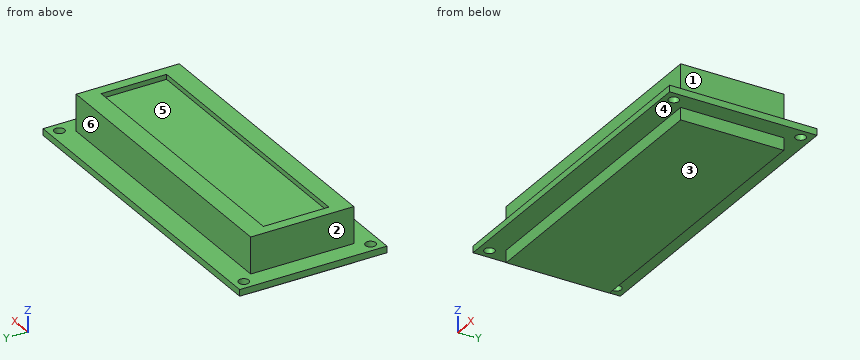
```python
from build123d import *

# Parameters (mm, degrees)
SKETCH2_W           = 80
SKETCH2_H           = 36
SKETCH2_W_2         = 71
SKETCH2_H_2         = 25.2
SKETCH2_W_3         = 66
SKETCH2_H_3         = 16
BOSS_EXTRUDE1_DEPTH = 1.6
BOSS_EXTRUDE2_START = 8.9
SKETCH2_3_W         = 71
SKETCH2_3_H         = 25.2
SKETCH2_3_W_2       = 66
SKETCH2_3_H_2       = 16
BOSS_EXTRUDE2_DEPTH = 13.5
CUT_EXTRUDE1_START  = 8.9
SKETCH2_4_W         = 66
SKETCH2_4_H         = 16
CUT_EXTRUDE1_DEPTH  = 1.2
SKETCH3_R           = 1.25
CUT_EXTRUDE2_DEPTH  = 45.757234052


with BuildPart() as part:
    # Sketch2 → Boss-Extrude1 (new body)
    # profile 1 of 3: a face of its own
    with BuildSketch(Plane.XY):
        Rectangle(SKETCH2_W, SKETCH2_H)
        Rectangle(SKETCH2_W_2, SKETCH2_H_2, mode=Mode.SUBTRACT)
    # profile 2 of 3: a face of its own
    with BuildSketch(Plane.XY):
        Rectangle(SKETCH2_W_2, SKETCH2_H_2)
        Rectangle(SKETCH2_W_3, SKETCH2_H_3, mode=Mode.SUBTRACT)
    # profile 3 of 3: a face of its own
    with BuildSketch(Plane.XY):
        Rectangle(SKETCH2_W_3, SKETCH2_H_3)
    extrude(amount=-BOSS_EXTRUDE1_DEPTH)

    # Sketch2<3> → Boss-Extrude2 (add)
    # profile 1 of 2: a face of its own
    with BuildSketch(Plane.XY.offset(BOSS_EXTRUDE2_START)):
        Rectangle(SKETCH2_3_W, SKETCH2_3_H)
        Rectangle(SKETCH2_3_W_2, SKETCH2_3_H_2, mode=Mode.SUBTRACT)
    # profile 2 of 2: a face of its own
    with BuildSketch(Plane.XY.offset(BOSS_EXTRUDE2_START)):
        Rectangle(SKETCH2_3_W_2, SKETCH2_3_H_2)
    extrude(amount=-BOSS_EXTRUDE2_DEPTH)

    # Sketch2<4> → Cut-Extrude1 (cut)
    with BuildSketch(Plane.XY.offset(CUT_EXTRUDE1_START)):
        Rectangle(SKETCH2_4_W, SKETCH2_4_H)
    extrude(amount=-CUT_EXTRUDE1_DEPTH, mode=Mode.SUBTRACT)

    # Sketch3 → Cut-Extrude2 (cut, through all)
    with BuildSketch(Plane.XY):
        with Locations((37.5, 15.5)):
            Circle(SKETCH3_R)
        with Locations((-37.5, 15.5)):
            Circle(SKETCH3_R)
        with Locations((37.5, -15.5)):
            Circle(SKETCH3_R)
        with Locations((-37.5, -15.5)):
            Circle(SKETCH3_R)
    extrude(amount=-CUT_EXTRUDE2_DEPTH, mode=Mode.SUBTRACT)


solid = part.part
```
Can you work these out from the model? Positions are in its coordinate system, mm. Face numbers are marked on the shaded views. A direction names the side the tool comes from. Round coordinates to 2 decimals unless told otherwise and drop trailing zeros. Order: outer loops, then holes, each group sorted by start corner. A loop starts at its lowest first (then second) coordinate and runs counter-clockwise, first axis right, second up.
(1) If I drill on L1, parallel to Y at x = -37.5, z = -0.45; L2, parallel to X at y = -4, z = 7.5; L3, parallel to Y at x = 24, z = 3, over which ranges is the centre line in solid material (lowest first)?
Results are:
L1: y = -18 to -16.75, -14.25 to 14.25, 16.75 to 18
L2: x = -35.5 to 35.5
L3: y = -12.6 to 12.6
(2) If we section it at C-C (y = -11.5): Please give me the cut outline in (x, z).
Results are:
outline: (-40, -1.6) - (-35.5, -1.6) - (-35.5, -4.6) - (35.5, -4.6) - (35.5, -1.6) - (40, -1.6) - (40, 0) - (35.5, 0) - (35.5, 8.9) - (-35.5, 8.9) - (-35.5, 0) - (-40, 0) - close
(3) We'd pull the mould along Y, two halves only. Please class the marked faces 4, 5 and 6: +Y half, -Y half, draft (parallel to the pull), parting line (faces both ways), or undercut.
Results are:
face 4: draft
face 5: undercut
face 6: +Y half
(4) I'm going to push flat-ended pins straight in: pin 1 (1.3 mm diameter, centred on x = 12, z = 8, fed in from -Y); pin 2 (5 mm diameter, centred on x = 1, y = 0.5, fed in from +Z); pin 3 (1.5 mm diameter, centred on y = 8, z = 6, fed in from -X); pin 4 (1.5 mm diameter, centred on x = -37.5, y = -15.5, fed in from -Z). Where does each tip first touch, or does it pass through?
Results are:
pin 1: stops at y = -12.6
pin 2: stops at z = 7.7
pin 3: stops at x = -35.5
pin 4: passes through
(5) If we section it at D-D (x = 6.5): Please give me the cut outline in (y, z).
Results are:
outline: (-18, -1.6) - (-12.6, -1.6) - (-12.6, -4.6) - (12.6, -4.6) - (12.6, -1.6) - (18, -1.6) - (18, 0) - (12.6, 0) - (12.6, 8.9) - (8, 8.9) - (8, 7.7) - (-8, 7.7) - (-8, 8.9) - (-12.6, 8.9) - (-12.6, 0) - (-18, 0) - close
(6) If we section it at B-B (y = 15.5): Please give me the cut outline in (x, z), plus the area to 3 significant figures.
Results are:
outline: (-40, -1.6) - (-38.75, -1.6) - (-38.75, 0) - (-40, 0) - close; (-36.25, -1.6) - (36.25, -1.6) - (36.25, 0) - (-36.25, 0) - close; (38.75, -1.6) - (40, -1.6) - (40, 0) - (38.75, 0) - close
area: 120 mm2
(7) On a 3-axis mill with a long thin cutter (end or side, diameter ignored), from which of +Z, -Z, +X, -X, +Y, -Y can I reach the whole of each face in a straight line? I mean the marked faces 1, 2 and 3. Say none if no direction works.
Results are:
face 1: +Z, +X, +Y, -Y
face 2: +Z, -X, +Y, -Y
face 3: -Z, +X, -X, +Y, -Y
(8) If we section it at A-A (x = -37.5): Please give me the cut outline in (y, z).
Results are:
outline: (-18, -1.6) - (-16.75, -1.6) - (-16.75, 0) - (-18, 0) - close; (-14.25, -1.6) - (14.25, -1.6) - (14.25, 0) - (-14.25, 0) - close; (16.75, -1.6) - (18, -1.6) - (18, 0) - (16.75, 0) - close
